```python
from build123d import *

# Parameters (mm, degrees)
LPATTERN1_COUNT     = 3
LPATTERN1_PITCH     = 24
LPATTERN2_COUNT     = 2
LPATTERN2_PITCH     = 24
BOSS_EXTRUDE1_REACH = 84.606
SKETCH4_W           = 24
SKETCH4_H           = 10
SKETCH5_W           = 10
SKETCH5_H           = 10
BOSS_EXTRUDE2_DEPTH = 10
CUT_EXTRUDE1_DEPTH  = 10
CHAMFER3_SIZE       = 2


with BuildPart() as part:
    # Sketch1 → Revolve1 (revolve)
    with BuildSketch(Plane(origin=(0, 0, 0), x_dir=(0, 0, -1), z_dir=(1, 0, 0))):
        Polygon((-12.875, 5), (-12.875, -5), (-6, -5), (-6, -3), (-10.875, -3), (-10.875, 5), align=None)
    revolve1 = revolve(axis=Axis((0, 27.077205882, 0), (0, -1, 0)))

    # LPattern1: Revolve1 ×3
    with Locations(*[(0, 0, -i * LPATTERN1_PITCH) for i in range(1, LPATTERN1_COUNT)]):
        add(revolve1)

    # LPattern2: Revolve1 ×2
    with Locations(*[(i * LPATTERN2_PITCH, 0, 0) for i in range(1, LPATTERN2_COUNT)]):
        add(revolve1)

    # LPattern2 copy 1 sketch → LPattern2 copy 1 (revolve)
    with BuildSketch(Plane(origin=(24, 0, -24), x_dir=(0, 0, -1), z_dir=(1, 0, 0))):
        Polygon((-12.875, 5), (-12.875, -5), (-6, -5), (-6, -3), (-10.875, -3), (-10.875, 5), align=None)
    revolve(axis=Axis((24, 27.077205882, -24), (0, -1, 0)))

    # LPattern2 copy 2 sketch → LPattern2 copy 2 (revolve)
    with BuildSketch(Plane(origin=(24, 0, -48), x_dir=(0, 0, -1), z_dir=(1, 0, 0))):
        Polygon((-12.875, 5), (-12.875, -5), (-6, -5), (-6, -3), (-10.875, -3), (-10.875, 5), align=None)
    revolve(axis=Axis((24, 27.077205882, -48), (0, -1, 0)))

    # Sketch4 → Boss-Extrude1 (add, up to next)
    with BuildSketch(Plane.XY.offset(12.875), mode=Mode.PRIVATE) as boss_extrude1_sk1:
        with Locations((12, 0)):
            Rectangle(SKETCH4_W, SKETCH4_H)
    boss_extrude1_tool1 = extrude(boss_extrude1_sk1.sketch, amount=-BOSS_EXTRUDE1_REACH, mode=Mode.PRIVATE) - part.part
    add(boss_extrude1_tool1.solids().sort_by_distance((12, 0, 12.875))[0])

    # Sketch5 → Boss-Extrude2 (add)
    with BuildSketch(Plane.XY.offset(12.875)):
        with Locations((12, 0)):
            Rectangle(SKETCH5_W, SKETCH5_H)
    extrude(amount=BOSS_EXTRUDE2_DEPTH)

    # Sketch8 → Cut-Extrude1 (cut)
    with BuildSketch(Plane.ZY.offset(-7)):
        Polygon((19.895725942, -3.5), (21.916451884, 0), (19.895725942, 3.5), (15.854274058, 3.5), (13.833548116, 0), (15.854274058, -3.5), align=None)
    extrude(amount=-CUT_EXTRUDE1_DEPTH, mode=Mode.SUBTRACT)

    # Chamfer3
    chamfer3_edges = [part.edges().sort_by_distance(p)[0] for p in [
        (12, -5, 22.875),
        (12, 5, 22.875),
    ]]
    chamfer(chamfer3_edges, length=CHAMFER3_SIZE)


solid = part.part
```
The listing builds one solid part. Answer for the finished solid, in the listing's coordinates (mm). A direction names the side the tool comes from. Round coordinates to 2 decimals unless told otherwise and drop trailing zeros. Loops run counter-clockwise (first coordinate to the right, second up) from the corner with the lowest first, then second, coordinate; pieces in that order, holes last.
1) Consider line 1 (Z direction, x = 0, y = -3.45) (3 decimals); line 2 (X direction, y = -4.5, z = 0) (3 decimals); line 3 (Z direction, x = 24, y = 2.75) (3 decimals). Determine where each line is inside the solid, lowest interval first.
Outcome:
line 1: z = -60.875 to -54, -42 to -30, -18 to -6, 6 to 12.875
line 2: x = -12.875 to -6, 6 to 18, 30 to 36.875
line 3: z = -60.875 to -58.875, -37.125 to -34.875, -13.125 to -10.875, 10.875 to 12.875
2) A cutting plane is placed at B-B on x = 1.5. Determine the outline of the cut face in (y, z) (3 decimals), plus the area to 3 significant figures.
Outcome:
outline: (-5, -60.787) - (5, -60.787) - (5, -58.771) - (-3, -58.771) - (-3, -53.809) - (-5, -53.809) - close; (-5, -42.191) - (-3, -42.191) - (-3, -37.229) - (5, -37.229) - (5, -34.771) - (-3, -34.771) - (-3, -29.809) - (-5, -29.809) - close; (-5, -18.191) - (-3, -18.191) - (-3, -13.229) - (5, -13.229) - (5, -10.771) - (-3, -10.771) - (-3, -5.809) - (-5, -5.809) - close; (-5, 5.809) - (-3, 5.809) - (-3, 10.771) - (5, 10.771) - (5, 12.875) - (-5, 12.875) - close
area: 150 mm2
3) Given P1, Ø1.5, axis at x = 0, z = -43.5, coming from the -Y side; P2, Ø3.5, axis at x = 3.5, y = 1.5, coming from the +Z side (3 decimals); P3, Ø5, axis at y = -4, z = -36.5, coming from the -X side; P4, Ø2, axis at x = 31.5, y = 4, coming from the -Z side, each flat-ended and moving along its own axis, determine where each tip first touches the part or whether it passes through.
Outcome:
P1: passes through
P2: stops at z = 12.875
P3: stops at x = -9.21
P4: stops at z = -59.11
4) A cutting plane is placed at D-D on z = -14. Determine the outline of the cut face in (x, y), plus the area to 3 significant figures.
Outcome:
outline: (-8.11, -5) - (8.11, -5) - (8.11, 5) - (4.27, 5) - (4.27, -3) - (-4.27, -3) - (-4.27, 5) - (-8.11, 5) - close; (15.89, -5) - (32.11, -5) - (32.11, 5) - (28.27, 5) - (28.27, -3) - (19.73, -3) - (19.73, 5) - (15.89, 5) - close
area: 188 mm2
5) A cutting plane is placed at C-C on y = 1.25. Give the number of separate pieces and of enclosed holes in the cut face, plus the area to 3 significant figures.
Outcome:
separate pieces: 2
enclosed holes: 8
area: 906 mm2
6) For faces 4 (the face through (20, 0, 12.875)), 5 (the face through (11.93, -1.726, 14.83)), 6 (the face through (-10.78, 1.06, -1.42)), determine the directions among +Z, -Z, +X, -X, +Y, -Y from which every point of the face is accessible in a straight line to the end or side of a thin tool.
Outcome:
face 4: +Z, +X, +Y, -Y
face 5: +X, -X
face 6: +Y
7) A cutting plane is placed at A-A on z = -2. Determine the outline of the cut face in (x, y).
Outcome:
outline: (-12.72, -5) - (-5.66, -5) - (-5.66, -3) - (-10.69, -3) - (-10.69, 5) - (-12.72, 5) - close; (5.66, -5) - (18.34, -5) - (18.34, -3) - (13.31, -3) - (13.31, 5) - (10.69, 5) - (10.69, -3) - (5.66, -3) - close; (29.66, -5) - (36.72, -5) - (36.72, 5) - (34.69, 5) - (34.69, -3) - (29.66, -3) - close
8) For a pull along Z with two mould halves and no side action, classify faces 1 (the face through (11.7, -5, -19.4)), 2 (the face through (11.93, -3.986, 21.889)), 3 (the face through (11.93, 1.774, 14.858)) as released by +Z, released by -Z, zero draft, split by the parting line, or undercut.
Outcome:
face 1: zero draft
face 2: released by +Z
face 3: undercut
